Geometry: final body of the model. Coordinates: model frame, mm. A direction names the side the tool comes from. Coordinates: 2 decimals unless noted, no trailing zeros. Order: outer loops, then holes, each group sorted by start corner. A loop starts at its lowest first (then second) coordinate and runs counter-clockwise, first axis right, second up. Notation, with made-up numbers: (81, 45) - (123, 45) arc R19 ccw to (123, 50) - close; hole circle Ø5 at (61.25, 62.25). An arc over 180 degrees is marked (long way). Use a Markdown table: item, result. Add a question column.
```python
from build123d import *

# Parameters (mm, degrees)
F0_R     = 2.25
F1_DEPTH = 5
F3_DEPTH = 8
F4_R     = 1.575
F5_DEPTH = 35.7601449816


with BuildPart() as f1:
    # F0 (on Front) → F1 (new body)
    with BuildSketch(Plane.XZ):
        Polygon((35.5, -3), (35.5, 3), (11.5355339059, 3), (8, -0.5355339059), (4.4644660941, 3), (-35.5, 3), (-35.5, -3), align=None)
        with Locations((-28.5, 0)):
            Circle(F0_R, mode=Mode.SUBTRACT)
        with Locations((28.5, 0)):
            Circle(F0_R, mode=Mode.SUBTRACT)
        Polygon((8, -0.5355339059), (11.5355339059, 3), (4.4644660941, 3), align=None)
        Polygon((4.4644660941, 3), (11.5355339059, 3), (8, 6.5355339059), align=None)
    extrude(amount=F1_DEPTH)

    # F2 (on face) → F3 (join)
    with BuildSketch(Plane.XZ.offset(5)):
        Polygon((11.5355339059, 3), (8, 6.5355339059), (4.4644660941, 3), (8, -0.5355339059), align=None)
    extrude(amount=F3_DEPTH)

    # F4 (on face) → F5 (cut, through all)
    with BuildSketch(Plane(origin=(4.267766953, 0, -4.267766953), x_dir=(0, 1, 0), z_dir=(0.7071067812, 0, -0.7071067812))):
        with Locations((-10.425, 7.7781745931)):
            Circle(F4_R)
    extrude(amount=-F5_DEPTH, mode=Mode.SUBTRACT)


solid = f1.part
```
1) Pin query (flat end, axial travel): pin 1 (1.5 mm diameter, centred on y = -8, z = -1.5, fed in from -X); pin 2 (6 mm diameter, centred on x = 12.5, y = -4.5, fed in from +Z); pin 3 (2.5 mm diameter, centred on x = 28.5, y = -3, fed in from +Z); pin 4 (4 mm diameter, centred on x = 13.5, z = 4, fed in from -Y). Return the tip coordinate at first contact, or that it passes through.
2) Draft query along Z for faces 6 (the face through (30.646, -2.465, 0.676)), 7 (the face through (0, -2, -3)), 8 (the face through (0, 0, 1)), 9 (the face through (-26.354, -2.465, 0.676)). Return one class per face: pulls with the +Z half, pulls with the -Z half, needs draft (parallel to the pull), parting line crosses it, or undercut.
3) Section B-B (x = -20.5). Return loops of the section in (y, z), then the cut area to 3 significant figures.
4) Section C-C (y = -6.75). Return loops of the section in (x, z).
5) Section A-A (x = -28.5). Return loops of the section in (y, z), then the cut area to 3 significant figures.
6) Ray query, line 1 along Z through (x, y) = (-28.5, -1.65); line 2 along X through (y, z) = (-3.5, -0.75); line 3 along Z through (x, y) = (-25.5, -0.5). Return the intervals inside material, ascending.
7) Set-up query: faces 1 (the face through (8.777, -11.586, 3.728)), 2 (the face through (9.743, -8.055, 1.207)), 3 (the face through (24, -2, 3)), 4 (the face through (-15, -2, 3)), 5 (the face through (6.207, -8.944, 1.257)). Return all of +Z, -Z, +X, -X, +Y, -Y with unobstructed straight access to the full face (end or side cutting, diameter ignored); none if empty.
Values follow:
| question | item | result |
|---|---|---|
| 1 | pin 1 | passes through |
| 1 | pin 2 | stops at z = 5.04 |
| 1 | pin 3 | stops at z = 3 |
| 1 | pin 4 | stops at y = -5 |
| 2 | face 6 | undercut |
| 2 | face 7 | pulls with the -Z half |
| 2 | face 8 | needs draft |
| 2 | face 9 | undercut |
| 3 | outline | (-5, -3) - (0, -3) - (0, 3) - (-5, 3) - close |
| 3 | area | 30.0 mm² |
| 4 | outline | (4.46, 3) - (8, -0.54) - (11.54, 3) - (8, 6.54) - close |
| 5 | outline | (-5, -3) - (0, -3) - (0, -2.25) - (-5, -2.25) - close; (-5, 2.25) - (0, 2.25) - (0, 3) - (-5, 3) - close |
| 5 | area | 7.50 mm² |
| 6 | line 1 | z = -3 to -2.25, 2.25 to 3 |
| 6 | line 2 | x = -35.5 to -30.62, -26.38 to 26.38, 30.62 to 35.5 |
| 6 | line 3 | z = -3 to 3 |
| 7 | face 1 | none |
| 7 | face 2 | -Z, +X, -Y |
| 7 | face 3 | +Z, +X, +Y, -Y |
| 7 | face 4 | +Z, -X, +Y, -Y |
| 7 | face 5 | -Z, -X, -Y |
